```python
from build123d import *

# Parameters (mm, degrees)
SKETCH1_W           = 7.069644311
SKETCH1_H           = 9.6
SKETCH1_R           = 2
SKETCH1_R_2         = 1.5
BOSS_EXTRUDE1_DEPTH = 2.5


with BuildPart() as part:
    # Sketch1 → Boss-Extrude1 (new, symmetric)
    # profile 1 of 9: a face of its own
    with BuildSketch(Plane(origin=(0, 0, 0), x_dir=(1, 0, 0), z_dir=(0, 1, 0))):
        with BuildLine():
            ThreePointArc((-45.466733516, 15.387532074), (-41.115924877, 24.768542983), (-34.856850116, 33))
            Line((-34.856850116, 33), (-45.466733516, 33))
            Line((-45.466733516, 33), (-45.466733516, 15.387532074))
        make_face()
    # profile 2 of 9: a face of its own
    with BuildSketch(Plane(origin=(0, 0, 0), x_dir=(1, 0, 0), z_dir=(0, 1, 0))):
        with BuildLine():
            Line((-33, 33), (-34.856850116, 33))
            ThreePointArc((-34.856850116, 33), (-41.115924877, 24.768542983), (-45.466733516, 15.387532074))
            Line((-45.466733516, 15.387532074), (-45.466733516, 13.267794591))
            Line((-45.466733516, 13.267794591), (-33, 13.267794591))
            Line((-33, 13.267794591), (-33, 33))
        make_face()
    # profile 3 of 9: a face of its own
    with BuildSketch(Plane(origin=(0, 0, 0), x_dir=(1, 0, 0), z_dir=(0, 1, 0))):
        with BuildLine():
            Line((-33, 0), (-33, 13.267794591))
            Line((-33, 13.267794591), (-45.466733516, 13.267794591))
            Line((-45.466733516, 13.267794591), (-45.466733516, -15.387532074))
            ThreePointArc((-45.466733516, -15.387532074), (-41.115924877, -24.768542983), (-34.856850116, -33))
            Line((-34.856850116, -33), (-31.966733516, -33))
            ThreePointArc((-31.966733516, -33), (-30.466733516, -31.5), (-28.966733516, -33))
            Line((-28.966733516, -33), (0, -33))
            ThreePointArc((0, -33), (-23.334523779, -23.334523779), (-33, 0))
        make_face()
    # profile 4 of 9: a face of its own
    with BuildSketch(Plane(origin=(0, 0, 0), x_dir=(1, 0, 0), z_dir=(0, 1, 0))):
        with BuildLine():
            Line((-34.856850116, -33), (-45.466733516, -33))
            Line((-45.466733516, -33), (-45.466733516, -47.472549547))
            Line((-45.466733516, -47.472549547), (-35.084874053, -47.472549547))
            ThreePointArc((-35.084874053, -47.472549547), (-33.206733516, -46.16), (-31.32859298, -47.472549547))
            Line((-31.32859298, -47.472549547), (-29.283755862, -47.472549547))
            Line((-29.283755862, -47.472549547), (-29.283755862, -42.6))
            Line((-29.283755862, -42.6), (-22.118770309, -42.6))
            ThreePointArc((-22.118770309, -42.6), (-28.889363626, -38.332814523), (-34.856850116, -33))
        make_face()
    # profile 5 of 9: a face of its own
    with BuildSketch(Plane(origin=(0, 0, 0), x_dir=(1, 0, 0), z_dir=(0, 1, 0))):
        with BuildLine():
            ThreePointArc((-34.856850116, -33), (-41.115924877, -24.768542983), (-45.466733516, -15.387532074))
            Line((-45.466733516, -15.387532074), (-45.466733516, -33))
            Line((-45.466733516, -33), (-34.856850116, -33))
        make_face()
    # profile 6 of 9: a face of its own
    with BuildSketch(Plane(origin=(0, 0, 0), x_dir=(1, 0, 0), z_dir=(0, 1, 0))):
        with BuildLine():
            Line((0, -42.6), (0, -33))
            Line((0, -33), (-28.966733516, -33))
            ThreePointArc((-28.966733516, -33), (-30.466733516, -34.5), (-31.966733516, -33))
            Line((-31.966733516, -33), (-34.856850116, -33))
            ThreePointArc((-34.856850116, -33), (-28.889363626, -38.332814523), (-22.118770309, -42.6))
            Line((-22.118770309, -42.6), (0, -42.6))
        make_face()
    # profile 7 of 9: a face of its own
    with BuildSketch(Plane(origin=(0, 0, 0), x_dir=(1, 0, 0), z_dir=(0, 1, 0))):
        with Locations((3.534822156, -37.8)):
            Rectangle(SKETCH1_W, SKETCH1_H)
    # profile 8 of 9: a face of its own
    with BuildSketch(Plane(origin=(0, 0, 0), x_dir=(1, 0, 0), z_dir=(0, 1, 0))):
        with BuildLine():
            ThreePointArc((11.216244138, -46.671145984), (18.757980211, -44.183007802), (25.786244138, -40.485424701))
            Line((25.786244138, -40.485424701), (25.786244138, -33))
            Line((25.786244138, -33), (7.069644311, -33))
            Line((7.069644311, -33), (7.069644311, -42.6))
            Line((7.069644311, -42.6), (11.216244138, -42.6))
            Line((11.216244138, -42.6), (11.216244138, -46.671145984))
        make_face()
    # profile 9 of 9: a face of its own
    with BuildSketch(Plane(origin=(0, 0, 0), x_dir=(1, 0, 0), z_dir=(0, 1, 0))):
        with BuildLine():
            Line((25.786244138, -107.999697871), (25.786244138, -40.485424701))
            ThreePointArc((25.786244138, -40.485424701), (18.757980211, -44.183007802), (11.216244138, -46.671145984))
            Line((11.216244138, -46.671145984), (11.216244138, -63.6))
            Line((11.216244138, -63.6), (-29.283755862, -63.6))
            Line((-29.283755862, -63.6), (-29.283755862, -47.472549547))
            Line((-29.283755862, -47.472549547), (-31.32859298, -47.472549547))
            ThreePointArc((-31.32859298, -47.472549547), (-31.237434013, -47.810916251), (-31.206733516, -48.16))
            ThreePointArc((-31.206733516, -48.16), (-33.555817265, -50.129299504), (-35.084874053, -47.472549547))
            Line((-35.084874053, -47.472549547), (-45.466733516, -47.472549547))
            Line((-45.466733516, -47.472549547), (-45.466733516, -107.999697871))
            Line((-45.466733516, -107.999697871), (25.786244138, -107.999697871))
        make_face()
        with Locations(Location((-30.463755862, -83, 0), (0, 0, 270))):
            Circle(SKETCH1_R, mode=Mode.SUBTRACT)
        with Locations(Location((-33.206733516, -58.04, 0), (0, 0, 270))):
            Circle(SKETCH1_R, mode=Mode.SUBTRACT)
        with Locations(Location((10.786244138, -83, 0), (0, 0, 270))):
            Circle(SKETCH1_R_2, mode=Mode.SUBTRACT)
        with Locations(Location((15.136244138, -58.04, 0), (0, 0, 270))):
            Circle(SKETCH1_R, mode=Mode.SUBTRACT)
        with Locations(Location((15.136244138, -48.16, 0), (0, 0, 270))):
            Circle(SKETCH1_R, mode=Mode.SUBTRACT)
    extrude(amount=BOSS_EXTRUDE1_DEPTH, both=True)


solid = part.part
```
Build history of the part. All positions in model axes, mm. A direction names the side the tool comes from. Round coordinates to 2 decimals unless told otherwise and drop trailing zeros. Write each loop counter-clockwise with the first axis right and the second up, starting at its lowest first coordinate (ties: lowest second). Pieces come first, ordered by that corner, then holes. Notation, with made-up numbers: (2.25, -17) - (20.25, -17) arc R28 cw to (20.25, 4) - close; hole circle Ø2 at (62.5, 55). An arc over 180 degrees is marked (long way). Write each question's results on one line, items separated by ' | '. Start each with the question number.
Item 1: Saw through at B-B (z = 83). Write the cut outline in (x, y), and give its area (3 significant figures).
Item 2: Saw through at D-D (z = 22.5). Write the cut outline in (x, y), and give its area (3 significant figures).
Item 3: Which spindle directions (+Z, -Z, +X, -X, +Y, -Y) get a long thin tool onto all of the face, cutting with end or side? Do faces 1 (the face through (-18, 2.5, 68)), 2 (the face through (13, 0, 33)), 3 (the face through (11.216, 0, 53)). Say none if no direction does.
Item 4: Wall check: L1, parallel to X at y = -0.85, z = 48.16; L2, parallel to X at y = 1.1, z = 83; L3, parallel to Z at x = 0.5, y = 0.4. Give the ranges that are in metal, low to high. Write a range as [from, to].
Item 5: Saw through at A-A (z = 58.04). Write the cut outline in (x, y), and give its area (3 significant figures).
Item 6: Drop flat-ended pins along their axis: P1, Ø4.5, axis at x = -33.21, z = 48.16, coming from the -Y side; P2, Ø3, axis at x = -30.46, z = 83, coming from the +Y side; P3, Ø1.5, axis at x = -18, y = 0, coming from the -Z side. Give the stop position or say it passes through.
Item 7: Saw through at C-C (y = 1.75). State how many separate pieces and enclosed holes the cut face has, and give its area (3 significant figures).
Item 8: Mould opens along X. For faces 4 (the face through (-18, -2.5, 68)), 5 (the face through (25.786, 0, 71)), 6 (the face through (-29.863, -0.035, 84.908)), 7 (the face through (-45.467, 0, 37)) say: pulls with the +X half, pulls with the -X half, needs draft (parallel to the pull), parting line crosses it, or undercut.
Results are:
1) outline: (-45.47, -2.5) - (-32.46, -2.5) - (-32.46, 2.5) - (-45.47, 2.5) - close; (-28.46, -2.5) - (9.29, -2.5) - (9.29, 2.5) - (-28.46, 2.5) - close; (12.29, -2.5) - (25.79, -2.5) - (25.79, 2.5) - (12.29, 2.5) - close | area: 321 mm²
2) outline: (-45.47, -2.5) - (-24.14, -2.5) - (-24.14, 2.5) - (-45.47, 2.5) - close | area: 107 mm²
3) face 1: +Z, -Z, +X, -X, +Y | face 2: -Z, +X, +Y, -Y | face 3: +Y, -Y
4) L1: x = [-45.47, -35.21], [-31.21, -29.28], [11.22, 13.14], [17.14, 25.79] | L2: x = [-45.47, -32.46], [-28.46, 9.29], [12.29, 25.79] | L3: z = [33, 42.6], [63.6, 108]
5) outline: (-45.47, -2.5) - (-35.21, -2.5) - (-35.21, 2.5) - (-45.47, 2.5) - close; (-31.21, -2.5) - (-29.28, -2.5) - (-29.28, 2.5) - (-31.21, 2.5) - close; (11.22, -2.5) - (13.14, -2.5) - (13.14, 2.5) - (11.22, 2.5) - close; (17.14, -2.5) - (25.79, -2.5) - (25.79, 2.5) - (17.14, 2.5) - close | area: 114 mm²
6) P1: stops at y = -2.5 | P2: passes through | P3: stops at z = 27.16
7) separate pieces: 1 | enclosed holes: 8 | area: 5,470 mm²
8) face 4: needs draft | face 5: pulls with the +X half | face 6: undercut | face 7: pulls with the -X half
